```python
from build123d import *

# Parameters (mm, degrees)
BOSS_EXTRUDE1_DEPTH = 25.4


with BuildPart() as part:
    # Sketch1 → Boss-Extrude1 (new body, symmetric)
    with BuildSketch(Plane.XY):
        Polygon((0, 496.697), (-50.8, 515.747), (-50.8, 101.6), (-101.6, 101.6), (-101.6, 0), (-76.2, 0), (-76.2, 76.2), (0, 76.2), (76.2, 76.2), (76.2, 0), (101.6, 0), (101.6, 101.6), (50.8, 101.6), (50.8, 515.747), align=None)
    extrude(amount=BOSS_EXTRUDE1_DEPTH, both=True)


solid = part.part
```
Geometry check sheet. Reference: the model listing, model coordinates, mm. A direction names the side the tool comes from. Give positions to 0.01 mm unless a question says otherwise; leave off trailing zeros. Loops run counter-clockwise (first coordinate to the right, second up) from the corner with the lowest first, then second, coordinate; pieces in that order, holes last. Notation, with made-up numbers: M 81.25,-39.5 L 117.25,-39.5 A27 cw 117.25,-16.5 Z; hole C -17,17 d3. An arc over 180 degrees is marked long. Write item = value, one per line. Start each with the question number.
1. Tool access check on faces 4 (the face through (77, 101.6, 0)), 5 (the face through (76.2, 39, 0)), 6 (the face through (25.756, 506.355, 0.356)). Record the directions out of +Z, -Z, +X, -X, +Y, -Y that give a thin tool (end or side, any length) a straight path to the whole face; none if there is none.
2. Section check C-C, the plane y = 326.5. Enter the section's corners in (x, z).
3. Thickness scan on probe 1 along X at (y, z) = (125, 22.5); probe 2 along X at (y, z) = (24.5, 8.5); probe 3 along Y at (x, z) = (89.5, -17.5). Record the ranges inside material, lowest first.
4. Section check A-A, the plane z = -1. Enter the section's corners in (x, y).
5. Go/stop test with flat-tipped pins: P1, Ø12, axis at x = -60, y = 378.5, coming from the +Z side; P2, Ø5, axis at x = -72, z = 13, coming from the +Y side; P3, Ø5, axis at x = -31, z = 3, coming from the +Y side; P4, Ø2, axis at y = 343.5, z = 6.5, coming from the -X side. Record where each tip stops, or that it passes through.
6. Draft check along X on faces 1 (the face through (101.6, 50, 0)), 2 (the face through (-1, 261, -25.4)), 3 (the face through (-1, 76.2, 0)). Enter one of: +X half, -X half, draft (parallel to the pull), parting line (faces both ways), or undercut.
7. Section check B-B, the plane x = -61.5. Enter the section's corners in (y, z).
Values follow:
q1.face_4 = +Z, -Z, +X, +Y
q1.face_5 = +Z, -Z, -Y
q1.face_6 = +Z, -Z, +Y
q2.outline = M -50.8,-25.4 L 50.8,-25.4 L 50.8,25.4 L -50.8,25.4 Z
q3.probe_1 = -50.8 to 50.8
q3.probe_2 = -101.6 to -76.2, 76.2 to 101.6
q3.probe_3 = 0 to 101.6
q4.outline = M -101.6,0 L -76.2,0 L -76.2,76.2 L 76.2,76.2 L 76.2,0 L 101.6,0 L 101.6,101.6 L 50.8,101.6 L 50.8,515.75 L 0,496.7 L -50.8,515.75 L -50.8,101.6 L -101.6,101.6 Z
q5.P1 = through
q5.P2 = 101.6
q5.P3 = 509.26
q5.P4 = -50.8
q6.face_1 = +X half
q6.face_2 = draft
q6.face_3 = undercut
q7.outline = M 76.2,-25.4 L 101.6,-25.4 L 101.6,25.4 L 76.2,25.4 Z
